Input: part model. Units: mm. Frame: model coordinates. A direction names the side the tool comes from. Round coordinates to 2 decimals unless told otherwise and drop trailing zeros. Order: outer loops, then holes, each group sorted by start corner. A loop starts at its lowest first (then second) coordinate and runs counter-clockwise, first axis right, second up. Notation, with made-up numbers: (21, 50.25) -> (45, 50.25) arc R5 ccw to (45, 58.25) -> close; hole circle Ø8 at (-16, -2.75). An arc over 180 degrees is marked (long way). Answer as CSV lines item,"result". Start each with the question number.
1) Section query C-C, the plane z = 17. Output: boundary loops of the cut face in (x, y), and give its area (3 significant figures).
2) Section query D-D, the plane z = 6.5. Output: boundary loops of the cut face in (x, y).
3) Section query A-A, the plane y = 0. Output: boundary loops of the cut face in (x, z).
4) Line query: L1, parallel to Z at x = 3.25, y = 0.5; L2, parallel to Y at x = 0, z = 16.5; L3, parallel to Y at x = 0.25, z = 5.5. Output: solid intervals per line, ascending.
5) Access query for faces 1 (the face through (2, -2, 0)), 2 (the face through (2, -2, 9)), 3 (the face through (-7.493, 0.33, 4.437)). Directions: +Z, -Z, +X, -X, +Y, -Y. A direction counts if a zero-diameter tool reaches every point of the face in a straight line with its end or side. Return the directions, or none.
6) First-contact query: P1, Ø3, axis at x = 3, z = -7, coming from the +Y side; P2, Ø4, axis at y = -2.5, z = -5, coming from the -X side; P3, Ø5, axis at y = -3, z = 1.5, coming from the -X side; P4, Ø2, axis at x = -4.5, z = 15.5, coming from the +Y side. Flat tips, straight axial feed; report the tip coordinate or a pass-through.
```python
from build123d import *

# Parameters (mm, degrees)
ESQUISSE1_R      = 7.5
EXTRUSION1_DEPTH = 9
ESQUISSE2_R      = 2
EXTRUSION2_DEPTH = 12
EXTRUSION3_START = 12
ESQUISSE3_R      = 2
EXTRUSION3_DEPTH = 12
CHANFREIN1_SIZE  = 0.4


with BuildPart() as part:
    # Esquisse1 → Extrusion1 (new body)
    with BuildSketch(Plane.XY):
        Circle(ESQUISSE1_R)
    extrude(amount=EXTRUSION1_DEPTH)

    # Esquisse2 → Extrusion2 (add)
    with BuildSketch(Plane.XY.offset(9)):
        Circle(ESQUISSE2_R)
    extrude(amount=EXTRUSION2_DEPTH)

    # Esquisse3 → Extrusion3 (add)
    with BuildSketch(Plane(origin=(0, 0, 0), x_dir=(-1, 0, 0), z_dir=(0, 0, -1)).offset(EXTRUSION3_START)):
        with Locations(Location((0, 0, 0), (0, 0, 180))):
            Circle(ESQUISSE3_R)
    extrude(amount=-EXTRUSION3_DEPTH)

    # Chanfrein1
    chanfrein1_edges = [part.edges().sort_by_distance(p)[0] for p in [
        (-2, 0, -12),
        (-2, 0, 21),
    ]]
    chamfer(chanfrein1_edges, length=CHANFREIN1_SIZE)


solid = part.part
```
Findings:
1,outline,"circle Ø4 at (0, 0)"
1,area,"12.6 mm^2"
2,outline,"circle Ø15 at (0, 0)"
3,outline,"(-7.5, 0) -> (-2, 0) -> (-2, -11.6) -> (-1.6, -12) -> (1.6, -12) -> (2, -11.6) -> (2, 0) -> (7.5, 0) -> (7.5, 9) -> (2, 9) -> (2, 20.6) -> (1.6, 21) -> (-1.6, 21) -> (-2, 20.6) -> (-2, 9) -> (-7.5, 9) -> close"
4,L1,"z = 0 to 9"
4,L2,"y = -2 to 2"
4,L3,"y = -7.5 to 7.5"
5,face 1,"-Z"
5,face 2,"+Z"
5,face 3,"+Z, -Z"
6,P1,"stops at y = 1.32"
6,P2,"stops at x = -1.94"
6,P3,"stops at x = -7.48"
6,P4,"passes through"
